from build123d import *

# Parameters (mm, degrees)
F0_W        = 63.5
F0_H        = 127
F1_DEPTH    = 31.75
F2_T        = -2.54
F3_T1_DEPTH = 88.9
F3_T3_DEPTH = 152.4


# Not quite as in the source:
# - a fillet or chamfer that OpenCascade refuses, or shapes differently, is made with other operations: its cross-section is extruded or revolved along the edge and cut away or added


with BuildPart() as f1:
    # F0 (on Front) → F1 (new body)
    with BuildSketch(Plane.XZ):
        Rectangle(F0_W, F0_H)
    extrude(amount=F1_DEPTH)

    # F2
    f2_openings = [f1.faces().sort_by_distance(p)[0] for p in [
        (0, -15.875, 63.5),
    ]]
    offset(amount=F2_T, openings=f2_openings)

    # F3: fillet of radius 5.08 on 4 edges, made by hand

    # F3_s2 → F3_t1 (cut)
    with BuildSketch(Plane.YZ.offset(-44.45)):
        with BuildLine():
            ThreePointArc((-31.75, 58.42), (-30.2621024484, 62.0121024484), (-26.67, 63.5))
            Line((-26.67, 63.5), (-31.75, 63.5))
            Line((-31.75, 63.5), (-31.75, 58.42))
        make_face()
        with BuildLine():
            ThreePointArc((-26.67, -63.5), (-30.2621024484, -62.0121024484), (-31.75, -58.42))
            Line((-31.75, -58.42), (-31.75, -63.5))
            Line((-31.75, -63.5), (-26.67, -63.5))
        make_face()
    extrude(amount=F3_T1_DEPTH, mode=Mode.SUBTRACT)

    # F3_s4 → F3_t3 (cut)
    with BuildSketch(Plane.XY.offset(-76.2)):
        with BuildLine():
            ThreePointArc((-31.75, -26.67), (-30.2621024484, -30.2621024484), (-26.67, -31.75))
            Line((-26.67, -31.75), (-31.75, -31.75))
            Line((-31.75, -31.75), (-31.75, -26.67))
        make_face()
        with BuildLine():
            ThreePointArc((31.75, -26.67), (30.2621024484, -30.2621024484), (26.67, -31.75))
            Line((26.67, -31.75), (31.75, -31.75))
            Line((31.75, -31.75), (31.75, -26.67))
        make_face()
    extrude(amount=F3_T3_DEPTH, mode=Mode.SUBTRACT)


solid = f1.part
For this review, take the finished solid that the model builds, in its own axes (mm). A direction names the side the tool comes from. Round coordinates to 2 decimals unless told otherwise and drop trailing zeros. Loops run counter-clockwise (first coordinate to the right, second up) from the corner with the lowest first, then second, coordinate; pieces in that order, holes last. Notation, with made-up numbers: (59.5, 39) - (86.5, 39) arc R21 ccw to (86.5, 46) - close; hole circle Ø9 at (86.25, -31.5). An arc over 180 degrees is marked (long way). Put each result on its own line as item: value. Start each with the question number.
1. Consider section A-A on z = -17.5. State the section outline as (x, y) points.
2. Consider section B-B on y = -7.5. State the section outline as (x, z) points.
3. Consider section C-C on x = 5.5. State the section outline as (y, z) points.
4. Mouldability with a two-part tool opening along X and no side actions: class faces 1 (the cylindrical face through (-30.301, -30.222, -0.889)), 2 (the cylindrical face through (30.301, -30.222, -0.889)), 3 (the flat face through (-29.21, -16, 0)), 4 (the cylindrical face through (-0.444, -30.222, -62.051)) as +X half, -X half, draft (parallel to the pull), parting line (faces both ways), or undercut.
5. For probe 1 along Y at (x, z) = (-15, 28); probe 2 along X at (y, z) = (-6, 19.5); probe 3 along Y at (x, z) = (-27.5, 25.5), list the stretches that pass through material, from the lowest coordinate up. Write a range as [from, to].
6. For faces 5 (the cylindrical face through (-0.44, -30.86, 61.29)), 6 (the flat face through (0, -2.54, 2)), list the 3-axis set-ups (+Z, -Z, +X, -X, +Y, -Y) from which the entire face can be reached by the end or side of a thin tool; tool diameter is ignored.
Result sheet:
1. outline: (-31.75, -26.67) arc R5.08 ccw to (-26.67, -31.75) - (26.67, -31.75) arc R5.08 ccw to (31.75, -26.67) - (31.75, 0) - (-31.75, 0) - close; hole (-29.21, -29.21) - (29.21, -29.21) - (29.21, -2.54) - (-29.21, -2.54) - close
2. outline: (-31.75, -63.5) - (31.75, -63.5) - (31.75, 63.5) - (29.21, 63.5) - (29.21, -60.96) - (-29.21, -60.96) - (-29.21, 63.5) - (-31.75, 63.5) - close
3. outline: (-31.75, -58.42) arc R5.08 ccw to (-26.67, -63.5) - (0, -63.5) - (0, 63.5) - (-2.54, 63.5) - (-2.54, -60.96) - (-29.21, -60.96) - (-29.21, 62.82) arc R5.08 ccw to (-31.75, 58.42) - close
4. face 1: -X half
4. face 2: +X half
4. face 3: undercut
4. face 4: draft
5. probe 1: [-31.75, -29.21], [-2.54, 0]
5. probe 2: [-31.75, -29.21], [29.21, 31.75]
5. probe 3: [-31.68, -29.21], [-2.54, 0]
6. face 5: +Z, +X, -X, -Y
6. face 6: +Z
